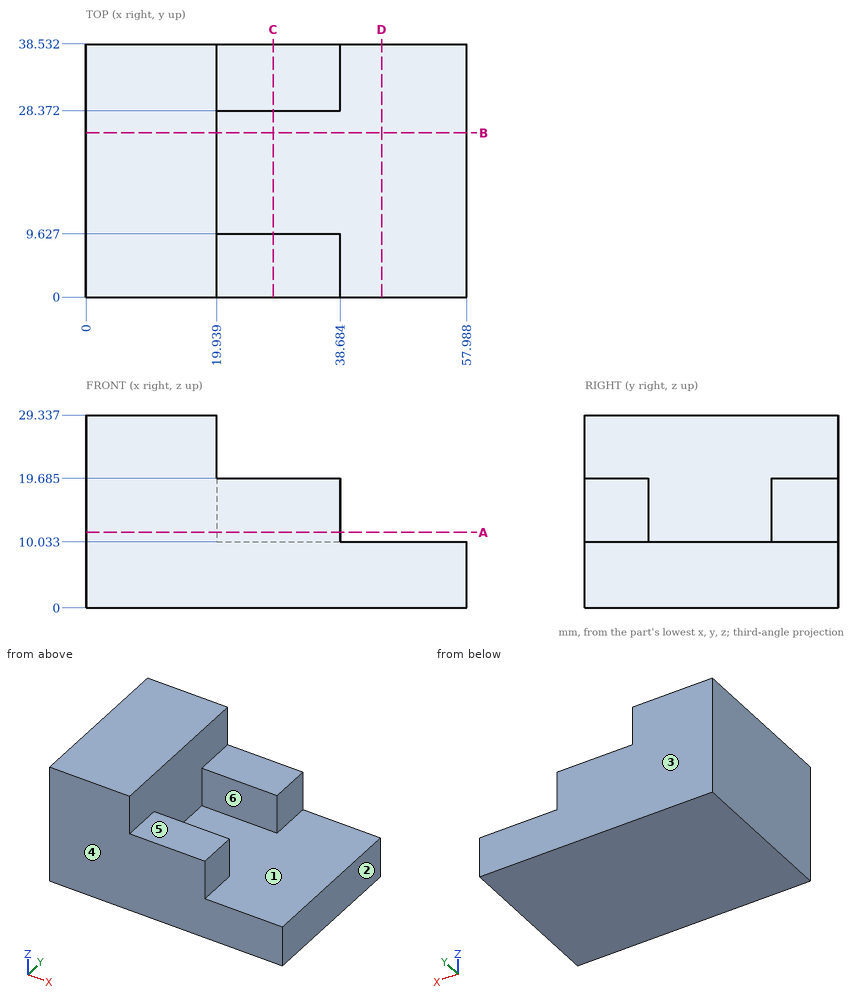
Design review of the part shown in the three views and the two pictorial views. Dimensions are in mm from the part's minimum x, y and z. A direction names the side the tool comes from. Give positions to 0.01 mm unless a question says otherwise; leave off trailing zeros. Loops run counter-clockwise (first coordinate to the right, second up) from the corner with the lowest first, then second, coordinate; pieces in that order, holes last. Notation, with made-up numbers: (-27.5, -19) -> (28.5, -19) arc R14 ccw to (28.5, 4) -> close; hole circle Ø6 at (78, -31). An arc over 180 degrees is marked (long way). Write each question's results on one line, items separated by ' | '.
1) Take a section at C-C, the plane x = 28.5. Give the boundary of the cut face in (y, z) (1 decimal).
Conclusion:
outline: (0, 0) -> (38.5, 0) -> (38.5, 19.7) -> (28.4, 19.7) -> (28.4, 10) -> (9.6, 10) -> (9.6, 19.7) -> (0, 19.7) -> close
2) Take a section at B-B, the plane y = 25. Give the boundary of the cut face in (x, z), plus the area to 3 significant figures.
Conclusion:
outline: (0, 0) -> (57.99, 0) -> (57.99, 10.03) -> (19.94, 10.03) -> (19.94, 29.34) -> (0, 29.34) -> close | area: 967 mm^2
3) Draft analysis for pull direction Y (two halves, no side actions). For the marked faces 1, 2 and 3, state which applies: pulls with the +Y half, pulls with the -Y half, needs draft (parallel to the pull), parting line crosses it, or undercut.
Conclusion:
face 1: undercut | face 2: needs draft | face 3: pulls with the +Y half
4) Take a section at A-A, the plane z = 11.5. Give the boundary of the cut face in (x, y) (1 decimal).
Conclusion:
outline: (0, 0) -> (38.7, 0) -> (38.7, 9.6) -> (19.9, 9.6) -> (19.9, 28.4) -> (38.7, 28.4) -> (38.7, 38.5) -> (0, 38.5) -> close
5) For line 1 along Y through (x, z) = (33, 18.75); line 2 along Z through (x, y) = (51.5, 12); line 3 along Z through (x, y) = (21, 4.5) (1 decimal), list the stretches that pass through material, from the lowest coordinate up. Write a range as from..to.
Conclusion:
line 1: y = 0..9.63, 28.37..38.53 | line 2: z = 0..10.03 | line 3: z = 0..19.7
6) Take a section at D-D, the plane x = 45. Give the boundary of the cut face in (y, z), plus the area to 3 significant figures.
Conclusion:
outline: (0, 0) -> (38.53, 0) -> (38.53, 10.03) -> (0, 10.03) -> close | area: 387 mm^2
7) Tool access review of the marked faces 4, 5 and 6: name each direction out of +Z, -Z, +X, -X, +Y, -Y from which nothing blocks a thin tool from reaching the whole face with its end or side.
Conclusion:
face 4: +Z, -Z, +X, -X, -Y | face 5: +Z, +X, +Y, -Y | face 6: +Z, +X
8) Insertion check: pin 1 Ø1 at (x, y) = (22, 28.5) entering from +Z (3 decimals); pin 2 Ø5 at (y, z) = (33, 14) entering from +X; pin 3 Ø1 at (y, z) = (32.5, 26.5) entering from +X. Each pin has a flat end and moves straight along its axis. Give the tip position at first contact, or say it passes through.
Conclusion:
pin 1: stops at z = 19.685 | pin 2: stops at x = 38.68 | pin 3: stops at x = 19.94
